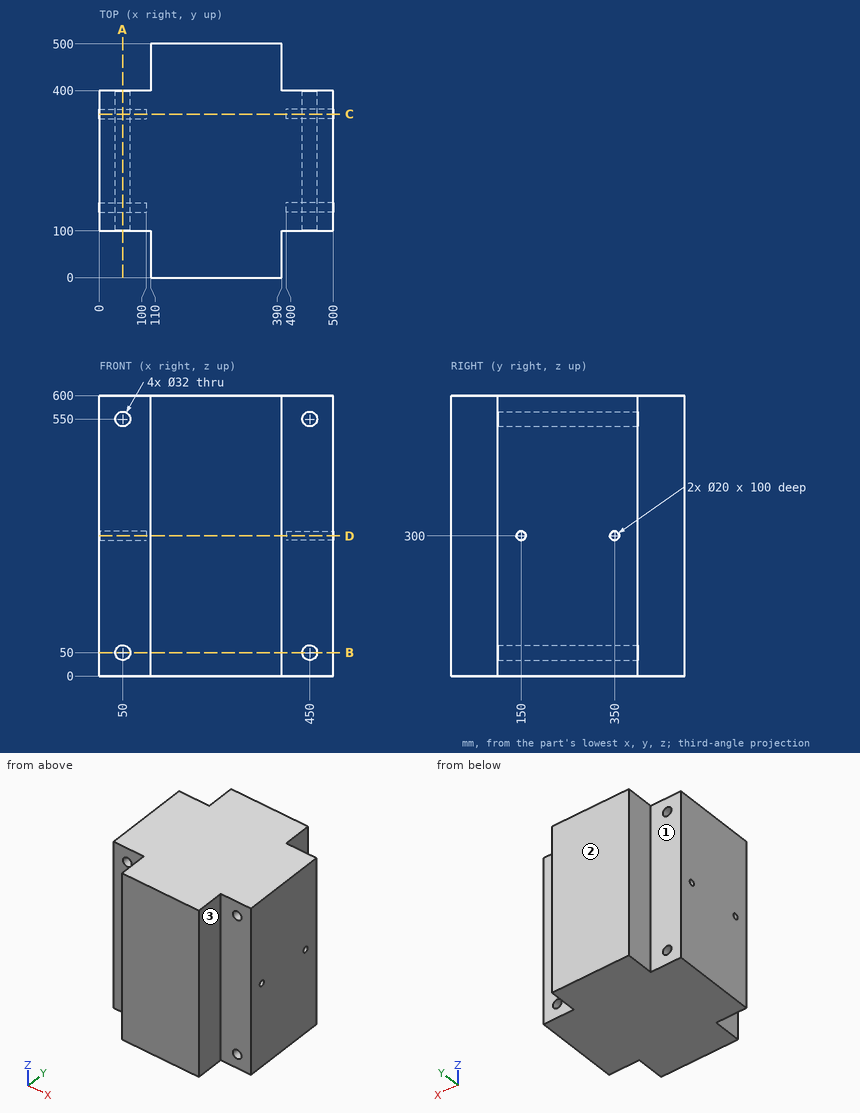
Geometry check sheet. Reference: drawing and pictorial views, mm from the part's lowest x, y, z. A direction names the side the tool comes from. Give positions to 0.01 mm unless a question says otherwise; leave off trailing zeros. Order: outer loops, then holes, each group sorted by start corner. A loop starts at its lowest first (then second) coordinate and runs counter-clockwise, first axis right, second up. Notation, with made-up numbers: (25, -4.5) -> (41, -4.5) arc R24 ccw to (41, 21.5) -> close; hole circle Ø2 at (77.25, 77.25). An arc over 180 degrees is marked (long way). Write each question's results on one line, items separated by ' | '. Start each with the question number.
(1) Sectioned sample at D-D (z = 300). Enter the section's corners in (x, y), plus the area to 3 significant figures.
(2) Sectioned sample at C-C (y = 350). Enter the section's corners in (x, z).
(3) Access from +Z, -Z, +X, -X, +Y, -Y to the whole of each face (thin tool, end or side, straight path). Record for the marked faces 1, 2 and 3.
(4) Sectioned sample at B-B (z = 50). Enter the section's corners in (x, y), plus the area to 3 significant figures.
(5) Scan lines: line 1 (Z direction, x = 451, y = 150); line 2 (Y direction, x = 70, z = 300); line 3 (Z direction, x = 450, y = 215). Record each from-to range of solid material in increasing order.
(6) Sectioned sample at A-A (x = 50). Enter the section's corners in (y, z).
(7) Gauge pin test, flat ends, axial feed: P1, Ø22, axis at y = 350, z = 299.5, coming from the +X side; P2, Ø3, axis at x = 448, z = 385.5, coming from the +Y side; P3, Ø18, axis at y = 350, z = 300, coming from the +X side; P4, Ø2, axis at y = 78.5, z = 90, coming from the -X side. Record the tip position at first contact, or that the pin passes through.
Answer below:
1) outline: (0, 100) -> (110, 100) -> (110, 0) -> (390, 0) -> (390, 100) -> (500, 100) -> (500, 140) -> (400, 140) -> (400, 160) -> (500, 160) -> (500, 340) -> (400, 340) -> (400, 360) -> (500, 360) -> (500, 400) -> (390, 400) -> (390, 500) -> (110, 500) -> (110, 400) -> (0, 400) -> (0, 360) -> (100, 360) -> (100, 340) -> (0, 340) -> (0, 160) -> (100, 160) -> (100, 140) -> (0, 140) -> close | area: 198,000 mm2
2) outline: (0, 0) -> (500, 0) -> (500, 290) -> (400, 290) -> (400, 310) -> (500, 310) -> (500, 600) -> (0, 600) -> (0, 310) -> (100, 310) -> (100, 290) -> (0, 290) -> close; hole circle Ø32 at (50, 50); hole circle Ø32 at (50, 550); hole circle Ø32 at (450, 50); hole circle Ø32 at (450, 550)
3) face 1: +Z, -Z, -X, +Y | face 2: +Z, -Z, +X, -X, +Y | face 3: +Z, -Z, +X, -Y
4) outline: (0, 100) -> (34, 100) -> (34, 400) -> (0, 400) -> close; (66, 100) -> (110, 100) -> (110, 0) -> (390, 0) -> (390, 100) -> (434, 100) -> (434, 400) -> (390, 400) -> (390, 500) -> (110, 500) -> (110, 400) -> (66, 400) -> close; (466, 100) -> (500, 100) -> (500, 400) -> (466, 400) -> close | area: 187,000 mm2
5) line 1: 0 to 34.03, 65.97 to 290, 310 to 534.03, 565.97 to 600 | line 2: 100 to 140, 160 to 340, 360 to 400 | line 3: 0 to 34, 66 to 534, 566 to 600
6) outline: (100, 0) -> (400, 0) -> (400, 34) -> (100, 34) -> close; (100, 66) -> (400, 66) -> (400, 534) -> (100, 534) -> close; (100, 566) -> (400, 566) -> (400, 600) -> (100, 600) -> close; hole circle Ø20 at (150, 300); hole circle Ø20 at (350, 300)
7) P1: x = 500 | P2: y = 400 | P3: x = 400 | P4: x = 110
